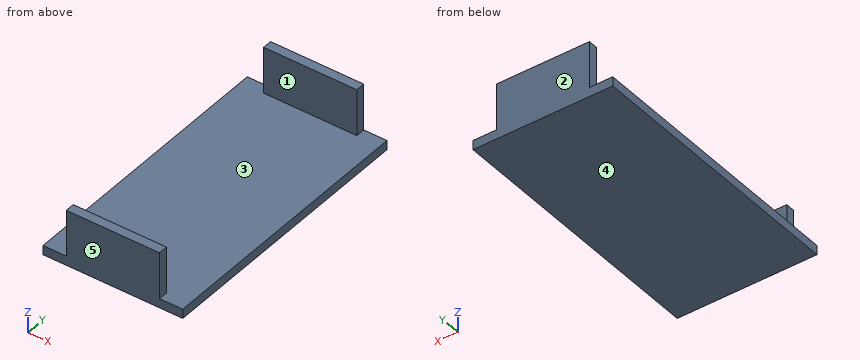
from build123d import *

# Parameters (mm, degrees)
SKETCH1_W           = 30
SKETCH1_H           = 59
BOSS_EXTRUDE1_DEPTH = 2
SKETCH2_W           = 20
SKETCH2_H           = 2
BOSS_EXTRUDE2_DEPTH = 10


with BuildPart() as part:
    # Sketch1 → Boss-Extrude1 (new body)
    with BuildSketch(Plane.XY):
        with Locations((15, 29.5)):
            Rectangle(SKETCH1_W, SKETCH1_H)
    extrude(amount=BOSS_EXTRUDE1_DEPTH)

    # Sketch2 → Boss-Extrude2 (add)
    with BuildSketch(Plane.XY.offset(2)):
        with Locations((15, 58)):
            Rectangle(SKETCH2_W, SKETCH2_H)
        with Locations((15, 1)):
            Rectangle(SKETCH2_W, SKETCH2_H)
    extrude(amount=BOSS_EXTRUDE2_DEPTH)


solid = part.part
Can you work these out from the model? Positions are in its coordinate system, mm. Face numbers are marked on the shaded views. A direction names the side the tool comes from. Coordinates: 2 decimals unless noted, no trailing zeros. Write each loop counter-clockwise with the first axis right and the second up, starting at its lowest first coordinate (ties: lowest second). Pieces come first, ordered by that corner, then holes. Notation, with made-up numbers: M 45,-32.75 L 93,-32.75 A13 ccw 93,-23.75 Z; hole C 16.5,28 d2. An arc over 180 degrees is marked long. Use one line per item in the form item = value.
Q1. If we section it at C-C (y = 29.5): Write out the boundary of the cut face in (x, z), then the cut area to 3 significant figures.
Model answer:
outline = M 0,0 L 30,0 L 30,2 L 0,2 Z
area = 60.0 mm^2
Q2. If we section it at A-A (z = 2.75): Write out the boundary of the cut face in (x, y).
Model answer:
outline = M 5,0 L 25,0 L 25,2 L 5,2 Z; M 5,57 L 25,57 L 25,59 L 5,59 Z
Q3. For P1, Ø3, axis at x = 11, y = 51.5, coming from the +Z side; P2, Ø0.6, axis at y = 1, z = 6.5, coming from the +X side; P3, Ø1.5, axis at y = 48, z = 4.5, coming from the +X side; P4, Ø1.6, axis at y = 58, z = 5, coming from the -X side, each with a flat end and sliding along its axis, tell me the tip position at first contact or that it passes through.
Model answer:
P1 = 2
P2 = 25
P3 = through
P4 = 5
Q4. We'd pull the mould along Y, two halves only. Please class the marked faces 3, 4 and 5: +Y half, -Y half, draft (parallel to the pull), parting line (faces both ways), or undercut.
Model answer:
face_3 = undercut
face_4 = draft
face_5 = -Y half
Q5. If we section it at B-B (x = 20.75): Write out the boundary of the cut face in (y, z), then the cut area to 3 significant figures.
Model answer:
outline = M 0,0 L 59,0 L 59,12 L 57,12 L 57,2 L 2,2 L 2,12 L 0,12 Z
area = 158 mm^2
Q6. I need wall thicknesses on line 1 along Y through (x, z) = (17.5, 8.75); line 2 along Z through (x, y) = (23, 17). Which ranges of each line are inside material? Lowest first, please. Write a range as from..to.
Model answer:
line_1 = 0..2, 57..59
line_2 = 0..2
Q7. For the marked faces 1 and 2, which set-ups out of +Z, -Z, +X, -X, +Y, -Y let a thin tool reach every point of the face, with its end or its side?
Model answer:
face_1 = +Z, +X, -X
face_2 = +Z, -Z, +X, -X, +Y
